Part model, mm, in its own coordinate system. A direction names the side the tool comes from. Give positions to 0.01 mm unless a question says otherwise; leave off trailing zeros. Write each loop counter-clockwise with the first axis right and the second up, starting at its lowest first coordinate (ties: lowest second). Pieces come first, ordered by that corner, then holes. Notation, with made-up numbers: (61, 61.25) - (116, 61.25) arc R27 cw to (116, 90.25) - close; hole circle Ø8 at (64, 49). An arc over 180 degrees is marked (long way). Answer as a JSON object with one key per item and string values. Group by question number.
```python
from build123d import *

# Parameters (mm, degrees)
F1_DEPTH = 45
F3_DEPTH = 40.5
F4_W     = 15
F4_H     = 10
F5_DEPTH = 30


with BuildPart() as f1:
    # F0 (on Front) → F1 (new body)
    with BuildSketch(Plane.XZ):
        Polygon((34.648232, 34.648232), (0, 0), (-34.648232, 34.648232), (0, 69.296465), (30.173114, 69.296465), (30.173114, 74.47869), (0, 104.651804), (-70.003571, 34.648232), (0, -35.355339), (70.003571, 34.648232), align=None)
    extrude(amount=F1_DEPTH)

    # F2 (on face) → F3 (cut)
    with BuildSketch(Plane.XZ.offset(45)):
        Polygon((-20.506097, 84.145707), (-49.497475, 55.154329), (-31.819805, 37.476659), (-2.828427, 66.468037), align=None)
        Polygon((-2.828427, 2.828427), (-31.819805, 31.819805), (-49.497475, 14.142136), (-20.506097, -14.849242), align=None)
        Polygon((31.819805, 31.819805), (2.828427, 2.828427), (20.506097, -14.849242), (49.497475, 14.142136), align=None)
    extrude(amount=-F3_DEPTH, mode=Mode.SUBTRACT)

    # F4 (on face) → F5 (cut)
    with BuildSketch(Plane(origin=(0, 0, 69.296465), x_dir=(1, 0, 0), z_dir=(0, 0, -1))):
        with Locations((15.086557, 25)):
            Rectangle(F4_W, F4_H)
    extrude(amount=-F5_DEPTH, mode=Mode.SUBTRACT)


solid = f1.part
```
1) Band-saw the part on A-A (y = -14.5). List the corners of the cut face in (x, z), plus the area to 3 significant figures.
2) Mould opens along Y. For faces 6 (the flat face through (15, -20, 80)), 7 (the flat face through (4, -45, 82)), 8 (the flat face through (-11.791, -25.034, -6.134)) say: pulls with the +Y half, pulls with the -Y half, needs draft (parallel to the pull), parting line crosses it, or undercut.
3) Band-saw the part on B-B (y = -23.5). List the corners of the cut face in (x, z), plus the area to 3 significant figures.
4) Which spindle directions (+Z, -Z, +X, -X, +Y, -Y) get a long thin tool onto all of the face, cutting with end or side? Do faces 1 (the flat face through (17, -4, 17)), 2 (the flat face through (26, -4.5, 9)), 3 (the flat face through (22.587, -25, 76)), 4 (the flat face through (7.587, -25, 83)), 5 (the flat face through (-11.54, -25.03, 75.18)). Say none if no direction does.
5) Drop flat-ended pins along their axis: P1, Ø12, axis at x = 12.5, z = 83, coming from the +Y side; P2, Ø14, axis at x = -25.5, z = 5, coming from the -Y side; P3, Ø9, axis at x = 8, y = -27.5, coming from the -Z side; P4, Ø8, axis at x = -54, y = -23.5, coming from the -Z side. Give the stop position or say it passes through.
6) Probe line 1 (Z direction, x = 3, y = -40); line 2 (Y direction, x = -31, z = 72.5); line 3 (Z direction, x = 7, y = -31). List the from-to ranges inside material, lowest first.
7) Band-saw the part on C-C (z = 9). List the corners of the cut face in (x, y).
8) Band-saw the part on D-D (z = 72.5). List the corners of the cut face in (x, y).
Verdict:
{
 "1": {"outline": "(-70, 34.65) - (-49.5, 14.14) - (-31.82, 31.82) - (-34.65, 34.65) - (-31.82, 37.48) - (-49.5, 55.15) - close; (-20.51, -14.85) - (0, -35.36) - (20.51, -14.85) - (2.83, 2.83) - (0, 0) - (-2.83, 2.83) - close; (-20.51, 84.15) - (-2.83, 66.47) - (0, 69.3) - (30.17, 69.3) - (30.17, 74.48) - (0, 104.65) - close; (31.82, 31.82) - (49.5, 14.14) - (70, 34.65) - (34.65, 34.65) - close", "area": "3,090 mm2"},
 "2": {"face 6": "undercut", "face 7": "pulls with the -Y half", "face 8": "needs draft"},
 "3": {"outline": "(-70, 34.65) - (-49.5, 14.14) - (-31.82, 31.82) - (-34.65, 34.65) - (-31.82, 37.48) - (-49.5, 55.15) - close; (-20.51, -14.85) - (0, -35.36) - (20.51, -14.85) - (2.83, 2.83) - (0, 0) - (-2.83, 2.83) - close; (-20.51, 84.15) - (-2.83, 66.47) - (0, 69.3) - (7.59, 69.3) - (7.59, 97.07) - (0, 104.65) - close; (22.59, 69.3) - (30.17, 69.3) - (30.17, 74.48) - (22.59, 82.07) - close; (31.82, 31.82) - (49.5, 14.14) - (70, 34.65) - (34.65, 34.65) - close", "area": "2,780 mm2"},
 "4": {"face 1": "+Y, -Y", "face 2": "-Y", "face 3": "+Z, -Z", "face 4": "+Z", "face 5": "-X, -Y"},
 "5": {"P1": "y = 0", "P2": "y = -4.5", "P3": "z = -31.86", "P4": "z = 14.64"},
 "6": {"line 1": "-32.36 to 2.66, 69.3 to 101.65", "line 2": "-4.5 to 0", "line 3": "-28.36 to -1.34, 69.3 to 97.65"},
 "7": {"outline": "(-44.36, -4.5) - (-9, -4.5) - (-9, 0) - (-44.36, 0) - close; (9, -4.5) - (44.36, -4.5) - (44.36, 0) - (9, 0) - close"},
 "8": {"outline": "(-32.15, -4.5) - (-8.86, -4.5) - (-8.86, -45) - (30.17, -45) - (30.17, 0) - (-32.15, 0) - close; hole (7.59, -30) - (22.59, -30) - (22.59, -20) - (7.59, -20) - close"}
}
